Check sheet for the modelled part. Datum: model origin and axes. Units: mm. A direction names the side the tool comes from. Coordinates: 2 decimals unless noted, no trailing zeros. Write each loop counter-clockwise with the first axis right and the second up, starting at its lowest first coordinate (ties: lowest second). Pieces come first, ordered by that corner, then holes. Notation, with made-up numbers: M -14.75,-35 L 9.25,-35 A14 ccw 9.25,-30 Z; hole C 60,-37 d10. An arc over 180 degrees is marked long. Answer as CSV lines item,"result".
from build123d import *

# Parameters (mm, degrees)
F0_W          = 50.8
F0_H          = 254
F0_H_2        = 50.8
F1_DEPTH      = 25.4
F2_W          = 863.6
F2_H          = 12.7
F2_H_2        = 25.4
F3_DEPTH      = 50.8
F3_DEPTH_BACK = 25.4


with BuildPart() as f1:
    # F0 (on Front) → F1 (new body)
    with BuildSketch(Plane.XZ):
        with Locations((0, -89.99076)):
            Rectangle(F0_W, F0_H)
        Polygon((-25.4, 37.00924), (25.4, 37.00924), (381, 37.00924), (381, 87.80924), (-381, 87.80924), (-381, 37.00924), align=None)
        with Locations((406.4, 62.40924)):
            Rectangle(F0_W, F0_H_2)
        with Locations((406.4, -89.99076)):
            Rectangle(F0_W, F0_H)
        with Locations((-406.4, -89.99076)):
            Rectangle(F0_W, F0_H)
        with Locations((-406.4, 62.40924)):
            Rectangle(F0_W, F0_H_2)
    extrude(amount=F1_DEPTH)

    # F2 (on face) → F3 (join, two sides)
    with BuildSketch(Plane.XZ.offset(25.4)) as f3_sk:
        with Locations((0, 94.15924)):
            Rectangle(F2_W, F2_H)
        with Locations((0, 75.10924)):
            Rectangle(F2_W, F2_H_2)
    extrude(amount=F3_DEPTH)
    extrude(f3_sk.sketch, amount=-F3_DEPTH_BACK)


solid = f1.part
1) Section check C-C, the plane y = -17.5. Record the boundary of the cut face in (x, z).
Answer key:
outline,"M -431.8,-216.99 L -381,-216.99 L -381,37.01 L -25.4,37.01 L -25.4,-216.99 L 25.4,-216.99 L 25.4,37.01 L 381,37.01 L 381,-216.99 L 431.8,-216.99 L 431.8,100.51 L -431.8,100.51 Z"
2) Section check B-B, the plane x = -316. Record the boundary of the cut face in (y, z).
Answer key:
outline,"M -76.2,62.41 L -25.4,62.41 L -25.4,37.01 L 0,37.01 L 0,100.51 L -76.2,100.51 Z"
3) Depth check by flat-ended pin: P1, Ø5, axis at x = -16, z = -171, coming from the -Y side; P2, Ø12.5, axis at x = 171.5, y = -12.5, coming from the -Z side; P3, Ø3, axis at x = 49.5, y = -34, coming from the -Z side. Enter the tip coordinate at first touch or a pass-through.
Answer key:
P1,"stops at y = -25.4"
P2,"stops at z = 37.01"
P3,"stops at z = 62.41"
4) Section check D-D, the plane y = -65. Record the boundary of the cut face in (x, z).
Answer key:
outline,"M -431.8,62.41 L 431.8,62.41 L 431.8,100.51 L -431.8,100.51 Z"
5) Mould release check, pull along X, two halves, no side actions. Record for faces 4 (the face through (-431.8, -22, -21)), 5 (the face through (381, -13, -92)), 6 (the face through (201, -13, 37.009)), 7 (the face through (-6, -76.2, 82)): pulls with the +X half, pulls with the -X half, needs draft (parallel to the pull), parting line crosses it, or undercut.
Answer key:
face 4,"pulls with the -X half"
face 5,"undercut"
face 6,"undercut"
face 7,"needs draft"
6) Section check A-A, the plane z = 17.5. Record the boundary of the cut face in (x, y).
Answer key:
outline,"M -431.8,-25.4 L -381,-25.4 L -381,0 L -431.8,0 Z; M -25.4,-25.4 L 25.4,-25.4 L 25.4,0 L -25.4,0 Z; M 381,-25.4 L 431.8,-25.4 L 431.8,0 L 381,0 Z"
7) Thickness scan on line 1 along X through (y, z) = (-5, -90); line 2 along Z through (x, y) = (23, -58); line 3 along Y through (x, z) = (-137, 38.5). Record the ranges inside material, lowest first.
Answer key:
line 1,"x = -431.8 to -381, -25.4 to 25.4, 381 to 431.8"
line 2,"z = 62.41 to 100.51"
line 3,"y = -25.4 to 0"
8) Tool access check on faces 1 (the face through (-25.4, -13, -92)), 2 (the face through (-2, -25.4, -25)), 3 (the face through (-407, -13, -216.991)). Record the directions out of +Z, -Z, +X, -X, +Y, -Y that give a thin tool (end or side, any length) a straight path to the whole face; none if there is none.
Answer key:
face 1,"-Z, +Y, -Y"
face 2,"-Z, +X, -X, -Y"
face 3,"-Z, +X, -X, +Y, -Y"
